Model file for the job. Use its own axes, mm. A direction names the side the tool comes from. Coordinates: 2 decimals unless noted, no trailing zeros. Order: outer loops, then holes, each group sorted by start corner. A loop starts at its lowest first (then second) coordinate and runs counter-clockwise, first axis right, second up. Notation, with made-up numbers: (19, 63) -> (30, 63) arc R24 ccw to (30, 74) -> close; hole circle Ø4 at (36, 40.25). An arc over 180 degrees is marked (long way). Write item = value, one per line. Start each with the question number.
Q1. Cut at A-A, the plane y = 108. List the corners of the cut face in (x, z).
Q2. Cut at B-B, the plane y = 48.5. List the corners of the cut face in (x, z).
Q3. Mould opens along Y. For faces 1 (the face through (24, 75, 6.35)), 2 (the face through (24.662, 132.693, 3.131)), 3 (the face through (37.99, 18.9, 3.13)) say: +Y half, -Y half, draft (parallel to the pull), parting line (faces both ways), or undercut.
Q4. 3-axis set-ups, long thin cutter, end or side, ignore diameter. For faces 4 (the face through (4.237, 25.148, 3.219)), 5 (the face through (34.453, 6.243, 3.219)), 6 (the face through (5.4, 69.73, 3.13)): which of +Z, -Z, +X, -X, +Y, -Y reach the whole face in a straight line?
Q5. Wall check: line 1 (Y direction, x = 8, z = 2.5); line 2 (X direction, y = 55, z = 5.75); line 3 (X direction, y = 135, z = 6.25). Give the ranges that are in metal, low to high. Write a range as from..to.
Q6. Cut at C-C, the plane y = 174. List the corners of the cut face in (x, z), plus the area to 3 significant figures.
Q7. Cut at D-D, the plane y = 129. List the corners of the cut face in (x, z), plus the area to 3 significant figures.
Q8. Flat gauge pins, fed straight in: pin 1 (3 mm diameter, centred on y = 105.5, z = 1.5, fed in from +X); pin 2 (2 mm diameter, centred on y = 140.5, z = 5.5, fed in from +X); pin 3 (1.9 mm diameter, centred on x = 23.5, z = 3, fed in from +Y); pin 4 (5 mm diameter, centred on x = 16.5, y = 157, fed in from +Z). Where does each tip first touch, or does it go through?
from build123d import *

# Parameters (mm, degrees)
BOSS_EXTRUDE1_DEPTH   = 6.35
CUT_EXTRUDE1_DEPTH    = 258.879971193
LPATTERN1_COUNT       = 9
LPATTERN1_PITCH       = 25.4
CUT_EXTRUDE2_DEPTH    = 258.879971193
LPATTERN3_START       = -252.481631985
LPATTERN3_OUTLINE_W   = 4.50356866
LPATTERN3_OUTLINE_H   = 6.35
LPATTERN3_DEPTH       = 52.327499141
LPATTERN3_START_2     = -187.454132844
LPATTERN3_2_OUTLINE_W = 4.50356866
LPATTERN3_2_OUTLINE_H = 6.35
LPATTERN3_2_DEPTH     = 12.7
LPATTERN3_START_3     = -162.054132844
LPATTERN3_3_OUTLINE_W = 4.50356866
LPATTERN3_3_OUTLINE_H = 6.35
LPATTERN3_3_DEPTH     = 12.7
LPATTERN3_START_4     = -136.654132844
LPATTERN3_4_OUTLINE_W = 4.50356866
LPATTERN3_4_OUTLINE_H = 6.35
LPATTERN3_4_DEPTH     = 12.7
LPATTERN3_START_5     = -111.254132844
LPATTERN3_5_OUTLINE_W = 4.50356866
LPATTERN3_5_OUTLINE_H = 6.35
LPATTERN3_5_DEPTH     = 12.7
LPATTERN3_START_6     = -85.854132844
LPATTERN3_6_OUTLINE_W = 4.50356866
LPATTERN3_6_OUTLINE_H = 6.35
LPATTERN3_6_DEPTH     = 12.7
LPATTERN3_START_7     = -60.454132844
LPATTERN3_7_OUTLINE_W = 4.50356866
LPATTERN3_7_OUTLINE_H = 6.35
LPATTERN3_7_DEPTH     = 12.7
LPATTERN3_START_8     = -35.054132844
LPATTERN3_8_OUTLINE_W = 4.50356866
LPATTERN3_8_OUTLINE_H = 6.35
LPATTERN3_8_DEPTH     = 12.7
LPATTERN3_START_9     = -225.661600657
LPATTERN3_9_OUTLINE_W = 2.832525799
LPATTERN3_9_OUTLINE_H = 6.35
LPATTERN3_9_DEPTH     = 13.028393953
SKETCH4_W             = 28.782231323
SKETCH4_H             = 17.896251878
CUT_EXTRUDE3_DEPTH    = 207.312084539
CUT_EXTRUDE4_DEPTH    = 194.552412762


# Read off the part's stored shape, not the designer's step: LPattern3
with BuildPart() as part:
    # Sketch1 → Boss-Extrude1 (new body)
    with BuildSketch(Plane.XY):
        Polygon((19.726920908, 254.76489438), (0, 0), (39.453841816, 0), align=None)
    extrude(amount=BOSS_EXTRUDE1_DEPTH)

    # Sketch2 → Cut-Extrude1 (cut, through all)
    with BuildSketch(Plane.XY.offset(6.35)):
        Polygon((0, 0), (0.98044984, 12.662097698), (5.4705779, 12.314418708), (4.490128061, -0.34767899), align=None)
    cut_extrude1 = extrude(amount=-CUT_EXTRUDE1_DEPTH, mode=Mode.SUBTRACT)

    # LPattern1: Cut-Extrude1 ×9
    with Locations(*[Vector(0.07720077476736964, 0.9970155667667973, 0) * (i * LPATTERN1_PITCH) for i in range(1, LPATTERN1_COUNT)]):
        add(cut_extrude1, mode=Mode.SUBTRACT)

    # Sketch3 → Cut-Extrude2 (cut, through all)
    with BuildSketch(Plane.XY.offset(6.35)):
        Polygon((39.453841816, 0), (38.473391976, 12.662097698), (33.983263916, 12.314418708), (34.963713756, -0.34767899), align=None)
    extrude(amount=-CUT_EXTRUDE2_DEPTH, mode=Mode.SUBTRACT)

    # LPattern3 outline → LPattern3 (cut)
    with BuildSketch(Plane(origin=(0, 0, 0), x_dir=(0.9970155667667971, 0.07720077476736921, 0), z_dir=(0.07720077476736921, -0.9970155667667973, 0)).offset(LPATTERN3_START)):
        with Locations((37.084310129, 3.175)):
            Rectangle(LPATTERN3_OUTLINE_W, LPATTERN3_OUTLINE_H)
    extrude(amount=LPATTERN3_DEPTH, mode=Mode.SUBTRACT)

    # LPattern3 2 outline → LPattern3 2 (cut)
    with BuildSketch(Plane(origin=(0, 0, 0), x_dir=(0.9970155667667971, 0.07720077476736921, 0), z_dir=(0.07720077476736921, -0.9970155667667973, 0)).offset(LPATTERN3_START_2)):
        with Locations((37.084310129, 3.175)):
            Rectangle(LPATTERN3_2_OUTLINE_W, LPATTERN3_2_OUTLINE_H)
    extrude(amount=LPATTERN3_2_DEPTH, mode=Mode.SUBTRACT)

    # LPattern3 3 outline → LPattern3 3 (cut)
    with BuildSketch(Plane(origin=(0, 0, 0), x_dir=(0.9970155667667971, 0.07720077476736921, 0), z_dir=(0.07720077476736921, -0.9970155667667973, 0)).offset(LPATTERN3_START_3)):
        with Locations((37.084310129, 3.175)):
            Rectangle(LPATTERN3_3_OUTLINE_W, LPATTERN3_3_OUTLINE_H)
    extrude(amount=LPATTERN3_3_DEPTH, mode=Mode.SUBTRACT)

    # LPattern3 4 outline → LPattern3 4 (cut)
    with BuildSketch(Plane(origin=(0, 0, 0), x_dir=(0.9970155667667971, 0.07720077476736921, 0), z_dir=(0.07720077476736921, -0.9970155667667973, 0)).offset(LPATTERN3_START_4)):
        with Locations((37.084310129, 3.175)):
            Rectangle(LPATTERN3_4_OUTLINE_W, LPATTERN3_4_OUTLINE_H)
    extrude(amount=LPATTERN3_4_DEPTH, mode=Mode.SUBTRACT)

    # LPattern3 5 outline → LPattern3 5 (cut)
    with BuildSketch(Plane(origin=(0, 0, 0), x_dir=(0.9970155667667971, 0.07720077476736921, 0), z_dir=(0.07720077476736921, -0.9970155667667973, 0)).offset(LPATTERN3_START_5)):
        with Locations((37.084310129, 3.175)):
            Rectangle(LPATTERN3_5_OUTLINE_W, LPATTERN3_5_OUTLINE_H)
    extrude(amount=LPATTERN3_5_DEPTH, mode=Mode.SUBTRACT)

    # LPattern3 6 outline → LPattern3 6 (cut)
    with BuildSketch(Plane(origin=(0, 0, 0), x_dir=(0.9970155667667971, 0.07720077476736921, 0), z_dir=(0.07720077476736921, -0.9970155667667973, 0)).offset(LPATTERN3_START_6)):
        with Locations((37.084310129, 3.175)):
            Rectangle(LPATTERN3_6_OUTLINE_W, LPATTERN3_6_OUTLINE_H)
    extrude(amount=LPATTERN3_6_DEPTH, mode=Mode.SUBTRACT)

    # LPattern3 7 outline → LPattern3 7 (cut)
    with BuildSketch(Plane(origin=(0, 0, 0), x_dir=(0.9970155667667971, 0.07720077476736921, 0), z_dir=(0.07720077476736921, -0.9970155667667973, 0)).offset(LPATTERN3_START_7)):
        with Locations((37.084310129, 3.175)):
            Rectangle(LPATTERN3_7_OUTLINE_W, LPATTERN3_7_OUTLINE_H)
    extrude(amount=LPATTERN3_7_DEPTH, mode=Mode.SUBTRACT)

    # LPattern3 8 outline → LPattern3 8 (cut)
    with BuildSketch(Plane(origin=(0, 0, 0), x_dir=(0.9970155667667971, 0.07720077476736921, 0), z_dir=(0.07720077476736921, -0.9970155667667973, 0)).offset(LPATTERN3_START_8)):
        with Locations((37.084310129, 3.175)):
            Rectangle(LPATTERN3_8_OUTLINE_W, LPATTERN3_8_OUTLINE_H)
    extrude(amount=LPATTERN3_8_DEPTH, mode=Mode.SUBTRACT)

    # LPattern3 9 outline → LPattern3 9 (cut)
    with BuildSketch(Plane(origin=(0, 0, 0), x_dir=(0.9970155667667971, 0.07720077476736921, 0), z_dir=(0.07720077476736921, -0.9970155667667973, 0)).offset(LPATTERN3_START_9)):
        with Locations((33.416262899, 3.175)):
            Rectangle(LPATTERN3_9_OUTLINE_W, LPATTERN3_9_OUTLINE_H)
    extrude(amount=LPATTERN3_9_DEPTH, mode=Mode.SUBTRACT)

    # Sketch4 → Cut-Extrude3 (cut, through all)
    with BuildSketch(Plane.XY.offset(6.35)):
        with Locations((18.872321894, 198.531912418)):
            Rectangle(SKETCH4_W, SKETCH4_H)
    extrude(amount=-CUT_EXTRUDE3_DEPTH, mode=Mode.SUBTRACT)

    # Sketch5 → Cut-Extrude4 (cut, through all)
    with BuildSketch(Plane.XY.offset(6.35)):
        Polygon((19.726920908, 114.176037685), (11.377749715, 6.35), (28.076092101, 6.35), align=None)
    extrude(amount=-CUT_EXTRUDE4_DEPTH, mode=Mode.SUBTRACT)


solid = part.part
Here are the results:
q1.outline = (12.88, 0) -> (19.25, 0) -> (19.25, 6.35) -> (12.88, 6.35) -> close; (20.21, 0) -> (26.57, 0) -> (26.57, 6.35) -> (20.21, 6.35) -> close
q2.outline = (3.76, 0) -> (14.64, 0) -> (14.64, 6.35) -> (3.76, 6.35) -> close; (24.81, 0) -> (35.7, 0) -> (35.7, 6.35) -> (24.81, 6.35) -> close
q3.face_1 = draft
q3.face_2 = undercut
q3.face_3 = +Y half
q4.face_4 = +Z, -Z
q4.face_5 = +Z, -Z, +X
q4.face_6 = +Z, -Z, -X, +Y
q5.line_1 = 0..50.33, 63.07..75.81, 88.55..101.28
q5.line_2 = 8.78..15.14, 24.31..30.68
q5.line_3 = 14.97..24.48
q6.outline = (13.47, 0) -> (25.98, 0) -> (25.98, 6.35) -> (13.47, 6.35) -> close
q6.area = 79.4 mm²
q7.outline = (14.51, 0) -> (24.95, 0) -> (24.95, 6.35) -> (14.51, 6.35) -> close
q7.area = 66.3 mm²
q8.pin_1 = 26.88
q8.pin_2 = 28.65
q8.pin_3 = 177.17
q8.pin_4 = 6.35
